Can you work these out from the drawing? Everything is in mm from the part's minimum corner. Round coordinates to 2 decimals unless told otherwise and drop trailing zeros. Write each loop counter-clockwise with the first axis right and the second up, starting at its lowest first coordinate (ties: lowest second). Pieces come first, ordered by that corner, then holes. Notation, with made-up numbers: (-18, 31.5) - (40, 31.5) arc R9 cw to (40, 41.5) - close; hole circle Ø5 at (49.5, 61.25). An arc over 180 degrees is marked (long way). One line per item, written item: value. Start each with the question number.
Item 1: Thinking about a two-plate mould opening in Y: for the marked faces 1 and 2, which applies, released by +Y, released by -Y, zero draft, split by the parting line, or undercut?
Item 2: If I drill on line 1 (X direction, y = 7.75, z = 22.5); line 2 (X direction, y = 11, z = 19.5), over which ranges is the centre line in solid material (lowest first)?
Item 3: Imagine slicing it at A-A, the plane x = 7.5. Please give me the cut outline in (y, z).
Item 4: For P1, Ø8, axis at x = 7.5, y = 7.5, coming from the -Z side; P2, Ø0.8, axis at x = 0.5, z = 6, coming from the +Y side; P3, Ø0.8, axis at x = 0.5, z = 33, coming from the -Y side; P4, Ø0.7, axis at x = 0.5, y = 5, coming from the +Z side, each with a flat end and sliding along its axis, tell me the tip position at first contact or that it passes through.
Item 5: Imagine slicing it at C-C, the plane x = 1.5. Please give me the cut outline in (y, z), then the cut area to 3 significant figures.
Item 6: Imagine slicing it at D-D, the plane z = 9. Please give me the cut outline in (x, y).
Item 7: Imagine slicing it at B-B, the plane y = 7.5. Please give me the cut outline in (x, z), then the cut area to 3 significant figures.
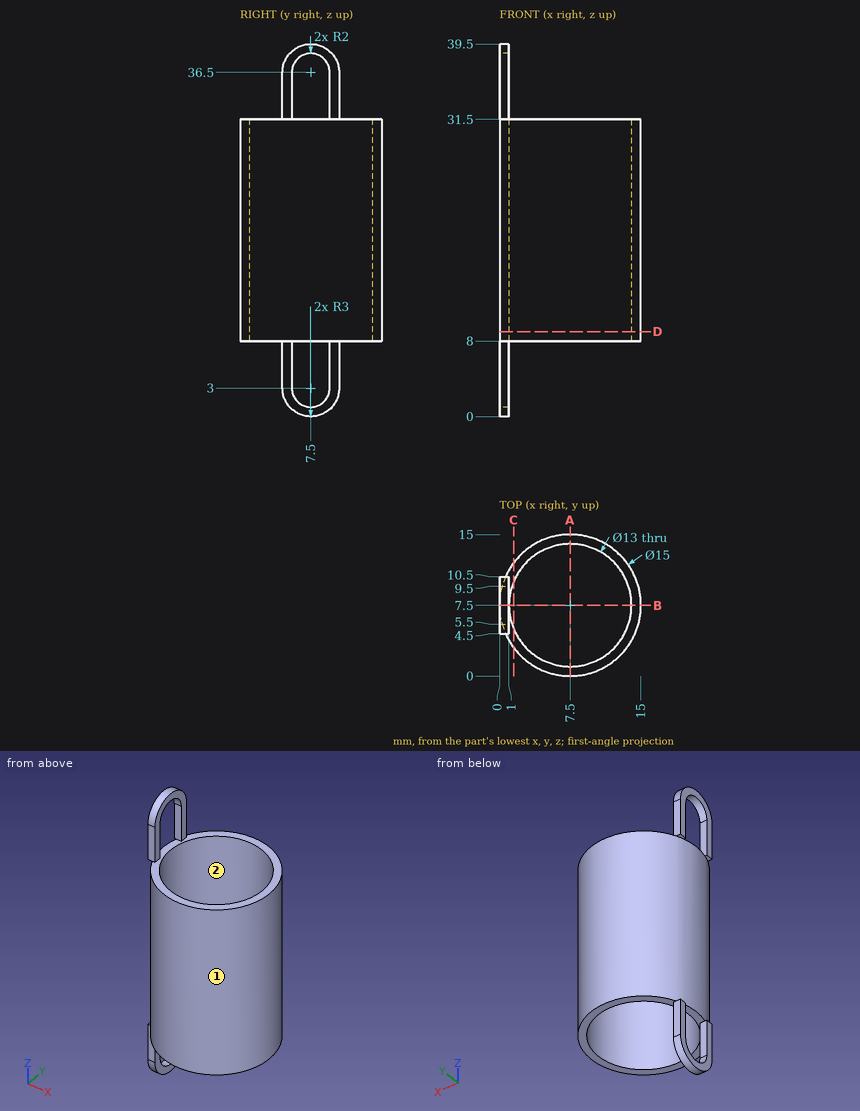
Values follow:
1. face 1: split by the parting line
1. face 2: undercut
2. line 1: x = 0 to 1, 14 to 15
2. line 2: x = 0.87 to 2.02, 12.98 to 14.13
3. outline: (0, 8) - (1, 8) - (1, 31.5) - (0, 31.5) - close; (14, 8) - (15, 8) - (15, 31.5) - (14, 31.5) - close
4. P1: passes through
4. P2: stops at y = 10.5
4. P3: stops at y = 4.5
4. P4: stops at z = 38.59
5. outline: (3, 8) - (5, 8) - (5, 31.5) - (3, 31.5) - close; (10, 8) - (12, 8) - (12, 31.5) - (10, 31.5) - close
5. area: 94.0 mm^2
6. outline: circle Ø15 at (7.5, 7.5); hole circle Ø13 at (7.5, 7.5)
7. outline: (0, 0) - (1, 0) - (1, 1) - (0, 1) - close; (0, 8) - (1, 8) - (1, 31.5) - (0, 31.5) - close; (0, 38.5) - (1, 38.5) - (1, 39.5) - (0, 39.5) - close; (14, 8) - (15, 8) - (15, 31.5) - (14, 31.5) - close
7. area: 49.0 mm^2
